Read the model definition and answer for the solid it produces. Units are mm, in the model's axes. Face numbers are marked on the shaded views. Coordinates: 2 decimals unless noted, no trailing zeros. Loops run counter-clockwise (first coordinate to the right, second up) from the corner with the lowest first, then second, coordinate; pieces in that order, holes last.
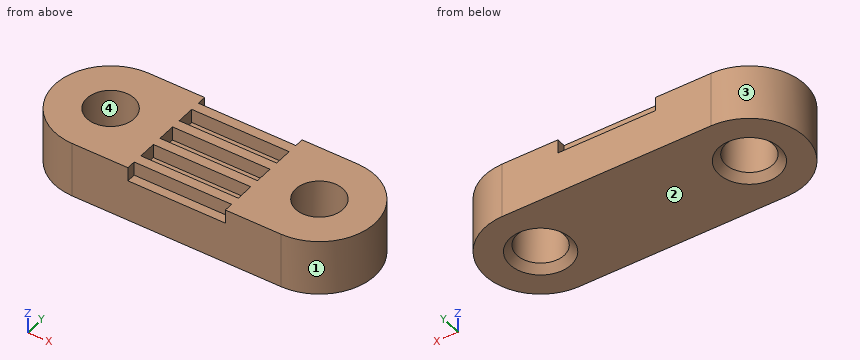
from build123d import *

# Parameters (mm, degrees)
SKETCH_R     = 1.7
PAD_DEPTH    = 4
SKETCH001_W  = 7
SKETCH001_H  = 1.3
POCKET_DEPTH = 1
CHAMFER_SIZE = 0.5


with BuildPart() as part:
    # Sketch → Pad (new body)
    with BuildSketch(Plane.XY):
        with BuildLine():
            ThreePointArc((-7.5, 4), (-11.5, 0), (-7.5, -4))
            Line((-7.5, -4), (7.5, -4))
            ThreePointArc((7.5, -4), (11.5, 0), (7.5, 4))
            Line((-7.5, 4), (7.5, 4))
        make_face()
        with Locations((-7.5, 0)):
            Circle(SKETCH_R, mode=Mode.SUBTRACT)
        with Locations((7.5, 0)):
            Circle(SKETCH_R, mode=Mode.SUBTRACT)
    extrude(amount=PAD_DEPTH)

    # Sketch001 → Pocket (cut)
    with BuildSketch(Plane.XY.offset(4)):
        with Locations((0, 2)):
            Rectangle(SKETCH001_W, SKETCH001_H)
        Rectangle(SKETCH001_W, SKETCH001_H)
        with Locations((0, -2)):
            Rectangle(SKETCH001_W, SKETCH001_H)
        with Locations((0, 4)):
            Rectangle(SKETCH001_W, SKETCH001_H)
        with Locations((0, -4)):
            Rectangle(SKETCH001_W, SKETCH001_H)
    extrude(amount=-POCKET_DEPTH, mode=Mode.SUBTRACT)

    # Chamfer
    chamfer_edges = [part.edges().sort_by_distance(p)[0] for p in [
        (-9.2, 0, 0),
        (5.8, 0, 0),
    ]]
    chamfer(chamfer_edges, length=CHAMFER_SIZE)


solid = part.part
Q1. Determine the mould class of the marked faces 1, 2, 3 and 4 for opening direction X: +X half, -X half, draft (parallel to the pull), parting line (faces both ways), or undercut.
Findings below:
face 1: +X half
face 2: draft
face 3: -X half
face 4: undercut
Q2. A cutting plane is placed at B-B (y = 0). Give the vertices of the cut face in (x, z), then the cut area to 3 significant figures.
Findings below:
outline: (-11.5, 0) - (-9.7, 0) - (-9.2, 0.5) - (-9.2, 4) - (-11.5, 4) - close; (-5.8, 0.5) - (-5.3, 0) - (5.3, 0) - (5.8, 0.5) - (5.8, 4) - (3.5, 4) - (3.5, 3) - (-3.5, 3) - (-3.5, 4) - (-5.8, 4) - close; (9.2, 0.5) - (9.7, 0) - (11.5, 0) - (11.5, 4) - (9.2, 4) - close
area: 57.3 mm2
Q3. Straight lines are drawn through the part: probe 1 along Y at (x, z) = (-7.5, 2.85); probe 2 along X at (y, z) = (-0.5, 1.1); probe 3 along X at (y, z) = (-0.75, 0.4). For each, find the intervals that lie inside material, in ascending order.
Findings below:
probe 1: y = -4 to -1.7, 1.7 to 4
probe 2: x = -11.47 to -9.12, -5.88 to 5.88, 9.12 to 11.47
probe 3: x = -11.43 to -9.14, -5.86 to 5.86, 9.14 to 11.43
Q4. A cutting plane is placed at A-A (z = 3.5). Give the vertices of the cut face in (x, y), then the cut area to 3 significant figures.
Findings below:
outline: (-7.5, -4) - (-3.5, -4) - (-3.5, -3.35) - (3.5, -3.35) - (3.5, -4) - (7.5, -4) arc R4 ccw to (7.5, 4) - (3.5, 4) - (3.5, 3.35) - (-3.5, 3.35) - (-3.5, 4) - (-7.5, 4) arc R4 ccw to start; hole circle Ø3.4 at (-7.5, 0); hole (-3.5, -2.65) - (3.5, -2.65) - (3.5, -1.35) - (-3.5, -1.35) - close; hole (-3.5, -0.65) - (3.5, -0.65) - (3.5, 0.65) - (-3.5, 0.65) - close; hole (-3.5, 1.35) - (3.5, 1.35) - (3.5, 2.65) - (-3.5, 2.65) - close; hole circle Ø3.4 at (7.5, 0)
area: 116 mm2
Q5. A cutting plane is placed at C-C (z = 2.15). Give the vertices of the cut face in (x, y).
Findings below:
outline: (-7.5, -4) - (7.5, -4) arc R4 ccw to (7.5, 4) - (-7.5, 4) arc R4 ccw to start; hole circle Ø3.4 at (-7.5, 0); hole circle Ø3.4 at (7.5, 0)
Q6. Flat-ended cylindrical pins translate along their axes: pin 1 Ø0.5 at (y, z) = (-2, 3.5) entering from +X; pin 2 Ø0.8 at (x, z) = (-1.5, 3.5) entering from -Y; pin 3 Ø1.5 at (x, y) = (-6.5, 1) entering from -Z; pin 4 Ø1.4 at (x, y) = (-1, 2) entering from +Z. Find the tip coordinate at first contact, or state that the pin passes through.
Findings below:
pin 1: stops at x = 11.1
pin 2: stops at y = -3.35
pin 3: stops at z = 0.04
pin 4: stops at z = 4
Q7. A cutting plane is placed at D-D (x = -1.75). Give the vertices of the cut face in (y, z).
Findings below:
outline: (-4, 0) - (4, 0) - (4, 3) - (3.35, 3) - (3.35, 4) - (2.65, 4) - (2.65, 3) - (1.35, 3) - (1.35, 4) - (0.65, 4) - (0.65, 3) - (-0.65, 3) - (-0.65, 4) - (-1.35, 4) - (-1.35, 3) - (-2.65, 3) - (-2.65, 4) - (-3.35, 4) - (-3.35, 3) - (-4, 3) - close
